```python
from build123d import *

# Parameters (mm, degrees)
SKETCH1_W             = 75
SKETCH1_H             = 75
BASE_DEPTH            = 7.5
SKETCH2_W             = 70
SKETCH2_H             = 70
SLOT_DEPTH            = 1.6
SKETCH3_W             = 67.858008496
SKETCH3_H             = 70
SLOT_COMPONENTS_DEPTH = 5.9


with BuildPart() as part:
    # Sketch1 → Base (new body)
    with BuildSketch(Plane(origin=(0, 0, 0), x_dir=(1, 0, 0), z_dir=(0, 1, 0))):
        Rectangle(SKETCH1_W, SKETCH1_H)
    extrude(amount=BASE_DEPTH)

    # Sketch2 → Slot (cut)
    with BuildSketch(Plane(origin=(0, 7.5, 0), x_dir=(1, 0, 0), z_dir=(0, 1, 0))):
        Rectangle(SKETCH2_W, SKETCH2_H)
    extrude(amount=-SLOT_DEPTH, mode=Mode.SUBTRACT)

    # Sketch3 → Slot-Components (cut)
    with BuildSketch(Plane(origin=(0, 5.9, 0), x_dir=(1, 0, 0), z_dir=(0, 1, 0))):
        Rectangle(SKETCH3_W, SKETCH3_H)
    extrude(amount=-SLOT_COMPONENTS_DEPTH, mode=Mode.SUBTRACT)


solid = part.part
```
Can you work these out from the model? Positions are in its coordinate system, mm. A direction names the side the tool comes from. Give positions to 0.01 mm unless a question says otherwise; leave off trailing zeros. Order: outer loops, then holes, each group sorted by start corner. A loop starts at its lowest first (then second) coordinate and runs counter-clockwise, first axis right, second up. Notation, with made-up numbers: M 54,57.25 L 87,57.25 A27 cw 87,96.25 Z; hole C 36,36 d2. An arc over 180 degrees is marked long. One line per item, written item: value.
1) On a 3-axis mill with a long thin cutter (end or side, diameter ignored), from which of +Z, -Z, +X, -X, +Y, -Y can I reach the whole of each face in a straight line? I mean faces 4 (the face through (-33.929, 3, 0)), 5 (the face through (35, 7, 0)), 6 (the face through (37.5, 4, 1)). Say none if no direction works.
Answer sheet:
face 4: +Y, -Y
face 5: +Y
face 6: +Z, -Z, +X, +Y, -Y
2) We'd pull the mould along Z, two halves only. Please class faces 1 (the face through (-1, 4, 37.5)), 2 (the face through (-35, 7, 0)), 3 (the face through (-1, 4, -37.5)): released by +Z, released by -Z, zero draft, split by the parting line, or undercut.
Answer sheet:
face 1: released by +Z
face 2: undercut
face 3: released by -Z
3) I want a section at A-A, the plane x = -0.5. List the corners of the cut face in (y, z) for me.
Answer sheet:
outline: M 0,-37.5 L 7.5,-37.5 L 7.5,-35 L 0,-35 Z; M 0,35 L 7.5,35 L 7.5,37.5 L 0,37.5 Z
4) I want a section at B-B, the plane z = 7.5. List the corners of the cut face in (x, y) for me.
Answer sheet:
outline: M -37.5,0 L -33.93,0 L -33.93,5.9 L -35,5.9 L -35,7.5 L -37.5,7.5 Z; M 33.93,0 L 37.5,0 L 37.5,7.5 L 35,7.5 L 35,5.9 L 33.93,5.9 Z
5) Please list where these lines run through material, in increasing order: line 1 along Z through (x, y) = (1.5, 1.75); line 2 along X through (y, z) = (0.75, -30).
Answer sheet:
line 1: z = -37.5 to -35, 35 to 37.5
line 2: x = -37.5 to -33.93, 33.93 to 37.5
6) I want a section at C-C, the plane y = 2.25. List the corners of the cut face in (x, z) for me.
Answer sheet:
outline: M -37.5,-37.5 L 37.5,-37.5 L 37.5,37.5 L -37.5,37.5 Z; hole M -33.93,-35 L 33.93,-35 L 33.93,35 L -33.93,35 Z
